The listing builds one solid part. Answer for the finished solid, in the listing's coordinates (mm). Face numbers are marked on the shaded views. A direction names the side the tool comes from. Coordinates: 2 decimals unless noted, no trailing zeros. Order: outer loops, then holes, each group sorted by start corner. A loop starts at its lowest first (then second) coordinate and runs counter-clockwise, first axis right, second up. Notation, with made-up numbers: (-10.5, 60.5) -> (42.5, 60.5) arc R32 ccw to (42.5, 90.5) -> close; hole circle Ø3 at (51, 84). An arc over 180 degrees is marked (long way). Write item = value, one per line.
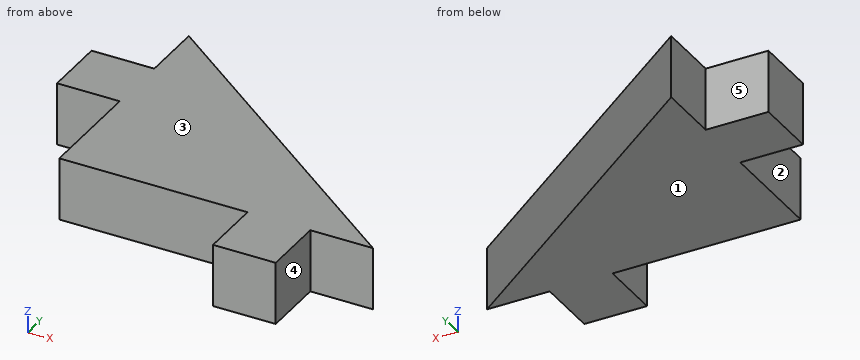
from build123d import *

# Parameters (mm, degrees)
SIDE_BOSS_EXTRUDE1_DEPTH               = 8
SKETCH2_W                              = 8
SKETCH2_H                              = 8
PUZZLE_SLOT_BACK_BOSS_EXTRUDE2_DEPTH   = 8
SKETCH3_W                              = 8
SKETCH3_H                              = 8
PUZZLE_SLOT_BOTTOM_BOSS_EXTRUDE3_DEPTH = 8


with BuildPart() as part:
    # Sketch1 → Side Boss-Extrude1 (new body)
    with BuildSketch(Plane.XY):
        Polygon((0, 0), (0, 30), (40, 0), align=None)
    extrude(amount=SIDE_BOSS_EXTRUDE1_DEPTH)

    # Sketch2 → Puzzle Slot Back Boss-Extrude2 (add)
    with BuildSketch(Plane.ZY):
        with Locations((4, 18)):
            Rectangle(SKETCH2_W, SKETCH2_H)
    extrude(amount=PUZZLE_SLOT_BACK_BOSS_EXTRUDE2_DEPTH)

    # Sketch3 → Puzzle Slot Bottom Boss-Extrude3 (add)
    with BuildSketch(Plane.XZ):
        with Locations((28, 4)):
            Rectangle(SKETCH3_W, SKETCH3_H)
    extrude(amount=PUZZLE_SLOT_BOTTOM_BOSS_EXTRUDE3_DEPTH)


solid = part.part
Q1. Each of these flat-tipped pins is pushed along its axis until it touches: pin 1 Ø2.5 at (x, z) = (-3, 4) entering from +Y; pin 2 Ø2.5 at (y, z) = (26, 3.5) entering from -X; pin 3 Ø4 at (x, z) = (25.5, 2.5) entering from +Y (3 decimals). Where does it stop, or does it pass through?
The answers:
pin_1 = 22
pin_2 = 0
pin_3 = 12.375
Q2. Find the intervals of material crossed by line 1 along Y through (x, z) = (-4.5, 1.5); line 2 along X through (y, z) = (-2, 6); line 3 along X through (y, z) = (24, 2.75), in increasing order.
The answers:
line_1 = 14 to 22
line_2 = 24 to 32
line_3 = 0 to 8
Q3. Section A-A, the plane z = 1.5 is taken. Give the vertices of the cut face in (x, y).
The answers:
outline = (-8, 14) -> (0, 14) -> (0, 0) -> (24, 0) -> (24, -8) -> (32, -8) -> (32, 0) -> (40, 0) -> (0, 30) -> (0, 22) -> (-8, 22) -> close
Q4. A tool of negligible diameter and unlimited length cuts with its end or side. For the marked faces 1, 2, 3, 4 and 5, from which of +Z, -Z, +X, -X, +Y, -Y can it reach the whole face along a straight path? Write none if from no direction.
The answers:
face_1 = -Z, +X, -X, +Y, -Y
face_2 = +Z, -Z, -X, -Y
face_3 = +Z, +X, -X, +Y, -Y
face_4 = +Z, -Z, +X, -Y
face_5 = +Z, -Z, -X, +Y
Q5. Section B-B, the plane y = -5 is taken. Give the vertices of the cut face in (x, z), plus the area to 3 significant figures.
The answers:
outline = (24, 0) -> (32, 0) -> (32, 8) -> (24, 8) -> close
area = 64.0 mm2
Q6. Section C-C, the plane x = -2.5 is taken. Give the vertices of the cut face in (y, z), plus the area to 3 significant figures.
The answers:
outline = (14, 0) -> (22, 0) -> (22, 8) -> (14, 8) -> close
area = 64.0 mm2
